Work out the finished part from the listing and answer in its coordinate system (mm). Face numbers are marked on the shaded views. A direction names the side the tool comes from. Give positions to 0.01 mm unless a question says otherwise; leave off trailing zeros. Order: outer loops, then holes, each group sorted by start corner. A loop starts at its lowest first (then second) coordinate and runs counter-clockwise, first axis right, second up.
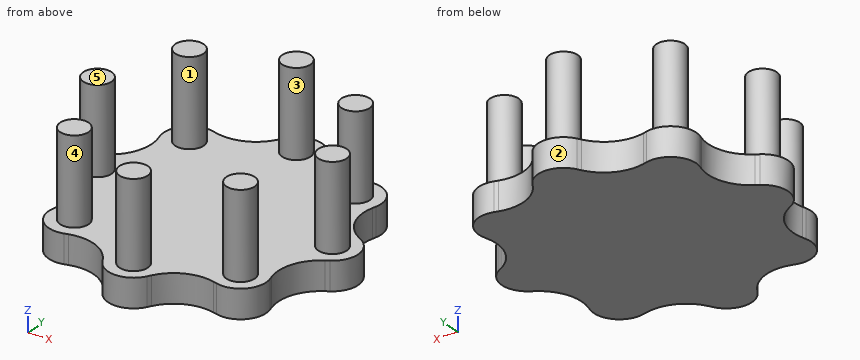
```python
from build123d import *

# Parameters (mm, degrees)
SKETCH2_R           = 25
PINION_DEPTH        = 200
PINION_BASE_DEPTH   = 50
CIRPATTERN1_COUNT   = 8
SKETCH1_R           = 180
BOSS_EXTRUDE1_DEPTH = 50
FILLET1_R           = 75


with BuildPart() as part:
    # Sketch2 → pinion (new body)
    with BuildSketch(Plane(origin=(0, 0, 0), x_dir=(0, 1, 0), z_dir=(0, 0, 1))):
        with Locations((-205, 0)):
            Circle(SKETCH2_R)
    extrude(amount=PINION_DEPTH)

    # Sketch2_3 → pinion base (add)
    with BuildSketch(Plane(origin=(0, 0, 0), x_dir=(0, 1, 0), z_dir=(0, 0, 1))):
        with BuildLine():
            Line((-227.5, 38.97114317), (-84.370095606, 121.607232002))
            Line((-84.370095606, 121.607232002), (-84.370095606, -121.607232002))
            Line((-84.370095606, -121.607232002), (-227.5, -38.97114317))
            ThreePointArc((-227.5, -38.97114317), (-250, 0), (-227.5, 38.97114317))
        make_face()
    extrude(amount=PINION_BASE_DEPTH)


with BuildPart() as cirpattern1_1:
    # CirPattern1: pattern copy
    add(part.part.rotate(Axis((0, 0, 0), (0, 0, 1)), 1 * 360 / CIRPATTERN1_COUNT))


with BuildPart() as cirpattern1_2:
    # CirPattern1: pattern copy
    add(part.part.rotate(Axis((0, 0, 0), (0, 0, 1)), 2 * 360 / CIRPATTERN1_COUNT))


with BuildPart() as cirpattern1_3:
    # CirPattern1: pattern copy
    add(part.part.rotate(Axis((0, 0, 0), (0, 0, 1)), 3 * 360 / CIRPATTERN1_COUNT))


with BuildPart() as cirpattern1_4:
    # CirPattern1: pattern copy
    add(part.part.rotate(Axis((0, 0, 0), (0, 0, 1)), 4 * 360 / CIRPATTERN1_COUNT))


with BuildPart() as cirpattern1_5:
    # CirPattern1: pattern copy
    add(part.part.rotate(Axis((0, 0, 0), (0, 0, 1)), 5 * 360 / CIRPATTERN1_COUNT))


with BuildPart() as cirpattern1_6:
    # CirPattern1: pattern copy
    add(part.part.rotate(Axis((0, 0, 0), (0, 0, 1)), 6 * 360 / CIRPATTERN1_COUNT))


with BuildPart() as cirpattern1_7:
    # CirPattern1: pattern copy
    add(part.part.rotate(Axis((0, 0, 0), (0, 0, 1)), 7 * 360 / CIRPATTERN1_COUNT))


with BuildPart() as part_1:
    add(part.part)

    add(cirpattern1_1.part)  # Boss-Extrude1 merges CirPattern1_1

    add(cirpattern1_2.part)  # Boss-Extrude1 merges CirPattern1_2

    add(cirpattern1_3.part)  # Boss-Extrude1 merges CirPattern1_3

    add(cirpattern1_4.part)  # Boss-Extrude1 merges CirPattern1_4

    add(cirpattern1_5.part)  # Boss-Extrude1 merges CirPattern1_5

    add(cirpattern1_6.part)  # Boss-Extrude1 merges CirPattern1_6

    add(cirpattern1_7.part)  # Boss-Extrude1 merges CirPattern1_7
    # Sketch1 → Boss-Extrude1 (add)
    with BuildSketch(Plane(origin=(0, 0, 0), x_dir=(0, 1, 0), z_dir=(0, 0, 1))):
        Circle(SKETCH1_R)
    extrude(amount=BOSS_EXTRUDE1_DEPTH)

    # Fillet1
    fillet1_edges = [part_1.edges().sort_by_distance(p)[0] for p in [
        (71.148381695, 171.767388028, 25),
        (171.767388028, 71.148381695, 25),
        (171.767388028, -71.148381695, 25),
        (71.148381695, -171.767388028, 25),
        (-71.148381695, -171.767388028, 25),
        (-171.767388028, -71.148381695, 25),
        (-171.767388028, 71.148381695, 25),
        (-71.148381695, 171.767388028, 25),
    ]]
    fillet(fillet1_edges, radius=FILLET1_R)


solid = part_1.part
```
1. Straight lines are drawn through the part: probe 1 along Y at (x, z) = (-1.5, 182.5); probe 2 along X at (y, z) = (145.5, 57); probe 3 along Y at (x, z) = (-109, 23). For each, find the intervals that lie inside material, in ascending order.
Findings below:
probe 1: y = -229.95 to -180.05, 180.05 to 229.95
probe 2: x = -169.95 to -119.96, 119.96 to 169.95
probe 3: y = -184.13 to 184.13
2. The part is cut by section A-A (x = 0). Write down the section's boundary in (y, z).
Findings below:
outline: (-250, 0) - (250, 0) - (250, 50) - (230, 50) - (230, 200) - (180, 200) - (180, 50) - (-180, 50) - (-180, 200) - (-230, 200) - (-230, 50) - (-250, 50) - close
3. Given P1, Ø12, axis at y = 152.5, z = 144.5, coming from the -X side; P2, Ø2, axis at x = 21, z = 101.5, coming from the -Y side; P3, Ø1, axis at y = -129.5, z = 166, coming from the +X side; P4, Ø5, axis at x = -156, y = -39.5, coming from the -Z side, each flat-ended and moving along its own axis, determine where each tip first touches the part or whether it passes through.
Findings below:
P1: stops at x = -169.91
P2: stops at y = -220
P3: stops at x = 164.99
P4: stops at z = 0
4. The part is cut by section D-D (x = -205). Write down the section's boundary in (y, z).
Findings below:
outline: (-55.39, 0) - (55.39, 0) - (55.39, 50) - (25, 50) - (25, 200) - (-25, 200) - (-25, 50) - (-55.39, 50) - close
5. The part is cut by section B-B (z = 188.5). Write down the section's boundary in (x, y), then the cut area to 3 significant figures.
Findings below:
outline: circle Ø50 at (-205, 0); circle Ø50 at (-144.96, -144.96); circle Ø50 at (-144.96, 144.96); circle Ø50 at (0, -205); circle Ø50 at (0, 205); circle Ø50 at (144.96, -144.96); circle Ø50 at (144.96, 144.96); circle Ø50 at (205, 0)
area: 15,700 mm2
6. Which of the six approach directions +Z, -Z, +X, -X, +Y, -Y give full straight-line access (tool end or side, diameter ignored) to the marked faces 1 and 2?
Findings below:
face 1: +Z
face 2: +Z, -Z, +Y
7. The mould has two halves that part along X. Classify the marked faces 3, 4 and 5: pulls with the +X half, pulls with the -X half, needs draft (parallel to the pull), parting line crosses it, or undercut.
Findings below:
face 3: parting line crosses it
face 4: undercut
face 5: needs draft
